Build history of the part. All positions in model axes, mm. Face numbers are marked on the shaded views. Give positions to 0.01 mm unless a question says otherwise; leave off trailing zeros. Write each loop counter-clockwise with the first axis right and the second up, starting at its lowest first coordinate (ties: lowest second). Pieces come first, ordered by that corner, then holes.
Autodesk Inventor part; units mm, degrees
ref_plane "YZ Plane" through (0, 0, 0) normal (1, 0, 0) x (0, 1, 0)
ref_plane "XZ Plane" through (0, 0, 0) normal (0, 1, 0) x (-1, 0, 0)
ref_plane "XY Plane" through (0, 0, 0) normal (0, 0, 1) x (1, 0, 0)
sketch "Sketch1" plane through (0, 0, 0) normal (0, 1, 0) x (-1, 0, 0)
  line L0 (-2, 2.5) -> (2, 2.5)
  line L1 (2, 2.5) -> (2, -2.5)
  line L2 (2, -2.5) -> (-2, -2.5)
  line L3 (-2, -2.5) -> (-2, 2.5)
  line L4 (-2, 2.5) -> (2, -2.5) construction
  line L5 (2, 2.5) -> (-2, -2.5) construction
  line L6 (0, 0) -> (2, 0) construction
  circle A0 centre (-0.5, 1.27) radius 0.825
  line L7 (-0.5, 1.27) -> (-0.5, 0) construction
  circle A1 centre (-0.5, -1.27) radius 0.825
  line L8 (-0.5, -1.27) -> (-0.5, 0) construction
  dimension "d0" = 4
  dimension "d1" = 5
  dimension "d3" = 1.65
  dimension "d4" = 1.27
  dimension "d5" = 1.5
extrude "Extrusion1" add sketch "Sketch1" along normal blind 3
sketch "Sketch2" plane through (0, 3, 0) normal (0, 1, 0) x (1, 0, 0)
  circle A0 centre (0.5, -1.27) radius 0.825
  circle A1 centre (0.5, -1.27) radius 0.965
  circle A2 centre (0.5, 1.27) radius 0.825
  circle A3 centre (0.5, 1.27) radius 0.965
  point P0 (0, 0)
  dimension "d8" = 1.93
  dimension "d9" = 1.93
extrude "Extrusion2" cut sketch "Sketch2" against normal blind 0.5
sketch "Sketch3" plane through (0, 3, 0) normal (0, 1, 0) x (1, 0, 0)
  line L0 (2, 2.5) -> (-2, 2.5)
  line L1 (-0.9, 2.5) -> (0.9, 2.5)
  line L2 (0.9, 2.5) -> (0.9, 5)
  line L3 (0.9, 5) -> (-0.9, 5)
  line L4 (-0.9, 5) -> (-0.9, 2.5)
  line L5 (-2, -2.5) -> (2, -2.5)
  line L6 (0, -2.5) -> (0, 2.5) construction
  point P0 (0, 0)
  dimension "d12" = 2.5
  dimension "d13" = 1.8
extrude "Extrusion3" add sketch "Sketch3" against normal up to surface (3 mm away)
sketch "Sketch4" plane through (0.9, 3, -2.5) normal (1, 0, 0) x (0, 0, -1)
  line L0 (2.2, 0) -> (2.2, -3) construction
  arc A0 (2.2, -3) -> (2.2, 0) centre (-2.5697, -1.5) ccw
  line L1 (2.5, 0) -> (2.5, -3)
  line L2 (2.2, 0) -> (2.5, 0)
  line L3 (2.5, 0) -> (2.5, -3)
  line L4 (2.5, -3) -> (2.2, -3)
  line L5 (2.5, -1.5) -> (1.25, -1.5) construction
  circle A1 centre (1.25, -1.5) radius 0.5
  point P0 (-2.5, -3)
  dimension "d16" = 5
  dimension "d17" = 0.3
  dimension "d18" = 1
  dimension "d19" = 1.25
extrude "Extrusion4" cut sketch "Sketch4" against normal blind 10
fillet "Fillet1" radius 0.5 2 edges at (0, 3, -4.7) (0, 0, -4.7)
fillet "Fillet2" radius 1 4 edges at (2, 1.5, -2.5) (2, 1.5, 2.5) (-2, 1.5, -2.5) (-2, 1.5, 2.5)
fillet "Fillet3" radius 0.2 18 edges at (2, 3, 0) (1.7071, 3, -2.2071) (0.95, 3, -2.5) (1.7071, 3, 2.2071) (0, 3, 2.5) (-1.7071, 3, 2.2071) (-2, 3, 0) (-1.7071, 3, -2.2071) (-0.95, 3, -2.5) (1.7071, 0, -2.2071) (0.95, 0, -2.5) (1.7071, 0, 2.2071) (0, 0, 2.5) (-1.7071, 0, 2.2071) (-2, 0, 0) (-1.7071, 0, -2.2071) (-0.95, 0, -2.5) (2, 0, 0)
equation "\"d9\" = d8"
properties part number "Camera_holder_PCB_1DOF"
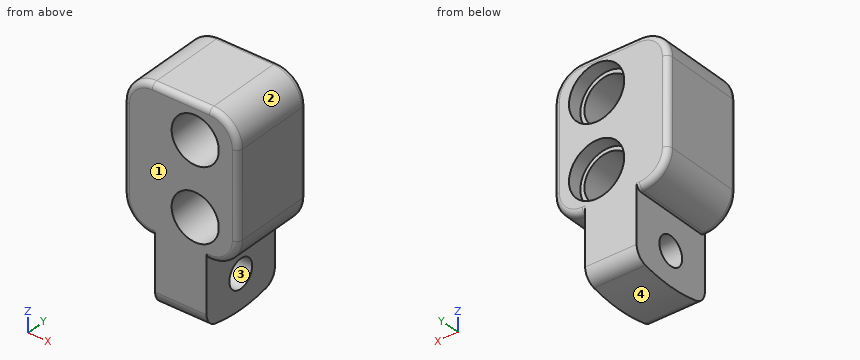
(1) Saw through at A-A, the plane x = 0.5. List the corners of the cut face in (y, z) (3 decimals), plus the area to 3 significant figures.
(2) Saw through at C-C, the plane y = 1.5. List the corners of the cut face in (x, z) (3 decimals).
(3) Mould opens along Y. For the marked faces 1, 2, 3 and 4 say: +Y half, -Y half, draft (parallel to the pull), parting line (faces both ways), or undercut.
(4) Drop a flat-ended pin along its axis: pin 1 (1.2 mm diameter, centred on x = 0.5, z = 1.27, fed in from +Y). Give the stop position or say it passes through.
(5) Probe line 1 (X direction, y = 1.35, z = -1.25); line 2 (Z direction, x = 1.2, y = 2.4); line 3 (Z direction, x = 0.45, y = 2.8). List the from-to ranges inside material, lowest first.
(6) Saw through at B-B, the plane z = -3.75. List the corners of the cut face in (x, y).
(7) Saw through at D-D, the plane x = -0.6. List the corners of the cut face in (y, z), plus the area to 3 significant figures.
Computed values:
1. outline: (0, -4.318) arc R0.5 ccw to (0.389, -4.805) arc R5 ccw to (2.611, -4.805) arc R0.5 ccw to (3, -4.318) - (3, -2.235) - (2.5, -2.235) - (2.5, -2.095) - (0, -2.095) - close; (0, -0.445) - (2.5, -0.445) - (2.5, -0.305) - (3, -0.305) - (3, 0.305) - (2.5, 0.305) - (2.5, 0.445) - (0, 0.445) - close; (0, 2.095) - (2.5, 2.095) - (2.5, 2.235) - (3, 2.235) - (3, 2.3) arc R0.2 ccw to (2.8, 2.5) - (0.2, 2.5) arc R0.2 ccw to (0, 2.3) - close; hole circle Ø1 at (1.5, -3.75)
1. area: 11.0 mm2
2. outline: (-2, -1.5) arc R1 ccw to (-1, -2.5) - (-0.9, -2.5) - (-0.9, -3.25) - (0.9, -3.25) - (0.9, -2.5) - (1, -2.5) arc R1 ccw to (2, -1.5) - (2, 1.5) arc R1 ccw to (1, 2.5) - (-1, 2.5) arc R1 ccw to (-2, 1.5) - close; (-0.9, -4.93) - (0.9, -4.93) - (0.9, -4.25) - (-0.9, -4.25) - close; hole circle Ø1.65 at (0.5, -1.27); hole circle Ø1.65 at (0.5, 1.27)
3. face 1: -Y half
3. face 2: draft
3. face 3: undercut
3. face 4: parting line
4. pin 1: passes through
5. line 1: x = -2 to -0.32, 1.32 to 2
5. line 2: z = -2.48 to -1.71, -0.83 to 0.83, 1.71 to 2.48
5. line 3: z = -4.72 to -2.23, -0.31 to 0.31, 2.23 to 2.5
6. outline: (-0.9, 0) - (0.9, 0) - (0.9, 1) - (-0.9, 1) - close; (-0.9, 2) - (0.9, 2) - (0.9, 3) - (-0.9, 3) - close
7. outline: (0, -4.32) arc R0.5 ccw to (0.39, -4.81) arc R5 ccw to (2.61, -4.81) arc R0.5 ccw to (3, -4.32) - (3, 2.3) arc R0.2 ccw to (2.8, 2.5) - (0.2, 2.5) arc R0.2 ccw to (0, 2.3) - close; hole circle Ø1 at (1.5, -3.75)
7. area: 21.2 mm2
